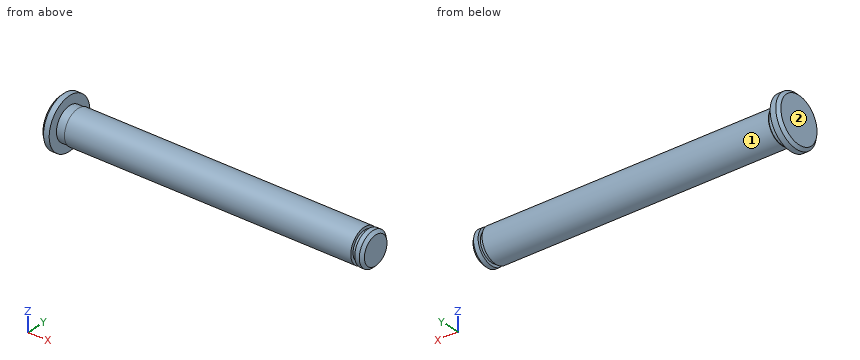
Autodesk Inventor part; units mm, degrees
ref_plane "pin_to_body_XY" through (1.5, 0, 0) normal (1, 0, 0) x (0, 0, -1)
ref_plane "pin_to_body_YZ" through (1.5, 0, 0) normal (0, 0, -1) x (0, 1, 0)
ref_plane "pin_to_body_ZX" through (1.5, 0, 0) normal (0, 1, 0) x (1, 0, 0)
sketch "Sketch_1" plane through (0, 0, 0) normal (0, 0, 1) x (1, 0, 0)
  line L0 (55.5, 0) -> (0, 0)
  line L1 (0, 0) -> (0, 4)
  line L2 (0, 4) -> (0.5, 4.5)
  line L3 (0.5, 4.5) -> (1.5, 4.5)
  line L4 (1.5, 4.5) -> (1.5, 2.9)
  line L5 (1.5, 2.9) -> (3, 2.9)
  line L6 (3, 2.9) -> (3, 3)
  line L7 (3, 3) -> (53.5, 3)
  line L8 (53.5, 3) -> (53.5, 2.5)
  line L9 (53.5, 2.5) -> (54.2, 2.5)
  line L10 (54.2, 2.5) -> (54.2, 3)
  line L11 (54.2, 3) -> (55, 3)
  line L12 (55, 3) -> (55.5, 2.5)
  line L13 (55.5, 2.5) -> (55.5, 0)
  line L14 (55.5, 0) -> (0, 0)
revolve "Revolution1" add sketch "Sketch_1" angle 360 about axis through (55.5, 0, 0) along (1, 0, 0)
ref_plane "pin_to_body_XY" through (1.5, 0, 0) normal (1, 0, 0) x (0, 0, -1)
ref_plane "pin_to_body_YZ" through (1.5, 0, 0) normal (0, 0, -1) x (0, 1, 0)
ref_plane "pin_to_body_ZX" through (1.5, 0, 0) normal (0, 1, 0) x (1, 0, 0)
ref_plane "pin_to_knuckle_XY" through (27.5, 0, 0) normal (-1, 0, 0) x (0, 0, -1)
ref_plane "pin_to_knuckle_YZ" through (27.5, 0, 0) normal (0, 0, -1) x (0, -1, 0)
ref_plane "pin_to_knuckle_ZX" through (27.5, 0, 0) normal (0, -1, 0) x (-1, 0, 0)
ref_plane "pin_to_rring_XY" through (53.85, 0, 0) normal (-1, 0, 0) x (0, 0, -1)
ref_plane "pin_to_rring_YZ" through (53.85, 0, 0) normal (0, 0, -1) x (0, -1, 0)
ref_plane "pin_to_rring_ZX" through (53.85, 0, 0) normal (0, -1, 0) x (-1, 0, 0)
properties part number "GSHCCGH6-52.0_D" material "ステンレス鋼"
Can you work these out from the model? Positions are in its coordinate system, mm. Face numbers are marked on the shaded views. A direction names the side the tool comes from. Give positions to 0.01 mm unless a question says otherwise; leave off trailing zeros. Write each loop counter-clockwise with the first axis right and the second up, starting at its lowest first coordinate (ties: lowest second). Pieces come first, ordered by that corner, then holes. Notation, with made-up numbers: (-31, 53) - (4, 53) arc R30 cw to (4, 88) - close; hole circle Ø4 at (4, 39.5). An arc over 180 degrees is marked (long way). Write item = value, one per line. Start each with the question number.
1. For pin 1 (4 mm diameter, centred on x = 7, y = 1.5, fed in from +Z); pin 2 (1 mm diameter, centred on x = 18, z = 1.5, fed in from +Y); pin 3 (1.5 mm diameter, centred on x = 10.5, y = -2.5, fed in from -Z), each with a flat end and sliding along its axis, tell me the tip position at first contact or that it passes through.
2. Imagine slicing it at C-C (x = 27.5). Please give me the cut outline in (y, z).
3. Please list where these lines run through material, in increasing order: line 1 (X direction, y = -0.75, z = -3.75); line 2 (Y direction, x = 40, z = 0.25).
4. Imagine slicing it at A-A (z = 0). Please give me the cut outline in (x, y), and give its area (3 significant figures).
5. On a 3-axis mill with a long thin cutter (end or side, diameter ignored), from which of +Z, -Z, +X, -X, +Y, -Y can I reach the whole of each face in a straight line? I mean the marked faces 1 and 2. Say none if no direction works.
Worked answers:
q1.pin_1 = 3
q1.pin_2 = 2.83
q1.pin_3 = -2.44
q2.outline = circle Ø6 at (0, 0)
q3.line_1 = 0 to 1.5
q3.line_2 = -2.99 to 2.99
q4.outline = (0, -4) - (0.5, -4.5) - (1.5, -4.5) - (1.5, -2.9) - (3, -2.9) - (3, -3) - (53.5, -3) - (53.5, -2.5) - (54.2, -2.5) - (54.2, -3) - (55, -3) - (55.5, -2.5) - (55.5, 2.5) - (55, 3) - (54.2, 3) - (54.2, 2.5) - (53.5, 2.5) - (53.5, 3) - (3, 3) - (3, 2.9) - (1.5, 2.9) - (1.5, 4.5) - (0.5, 4.5) - (0, 4) - close
q4.area = 336 mm2
q5.face_1 = +X
q5.face_2 = +Z, -Z, -X, +Y, -Y
